Could you check a few things on this drawing? It's one solid part, dimensions in mm from its lowest x, y, z. Coordinates: 2 decimals unless noted, no trailing zeros. Loops run counter-clockwise (first coordinate to the right, second up) from the corner with the lowest first, then second, coordinate; pieces in that order, holes last.
1) Imagine slicing it at B-B on z = 5. Please give me the cut outline in (x, y) (1 decimal).
2) If I drill on line 1 along X through (y, z) = (4.85, 25); line 2 along X through (y, z) = (3.05, 27); line 3 along Z through (x, y) = (44, 1.55) (1 decimal), over which ranges is the centre line in solid material (lowest first)?
3) Will these pins go through, and if not, where does the flat tip stop? P1, Ø6, axis at x = 44, z = 27, coming from the +Y side; P2, Ø6, axis at x = 43, z = 27.71, coming from the +Y side; P3, Ø1, axis at x = 30.5, y = 1, coming from the -Z side; P4, Ø2.5, axis at y = 3, z = 29.5, coming from the -X side (3 decimals).
4) Imagine slicing it at C-C on y = 3. Please give me the cut outline in (x, z), plus the area to 3 significant figures.
5) Imagine slicing it at A-A on x = 43. Please give me the cut outline in (y, z), plus the area to 3 significant figures.
6) Thinking about a two-plate mould opening in X: for the marked faces 1, 2 and 3, which applies, released by +X, released by -X, zero draft, split by the parting line, or undercut?
7) Imagine slicing it at D-D on x = 28. Please give me the cut outline in (y, z).
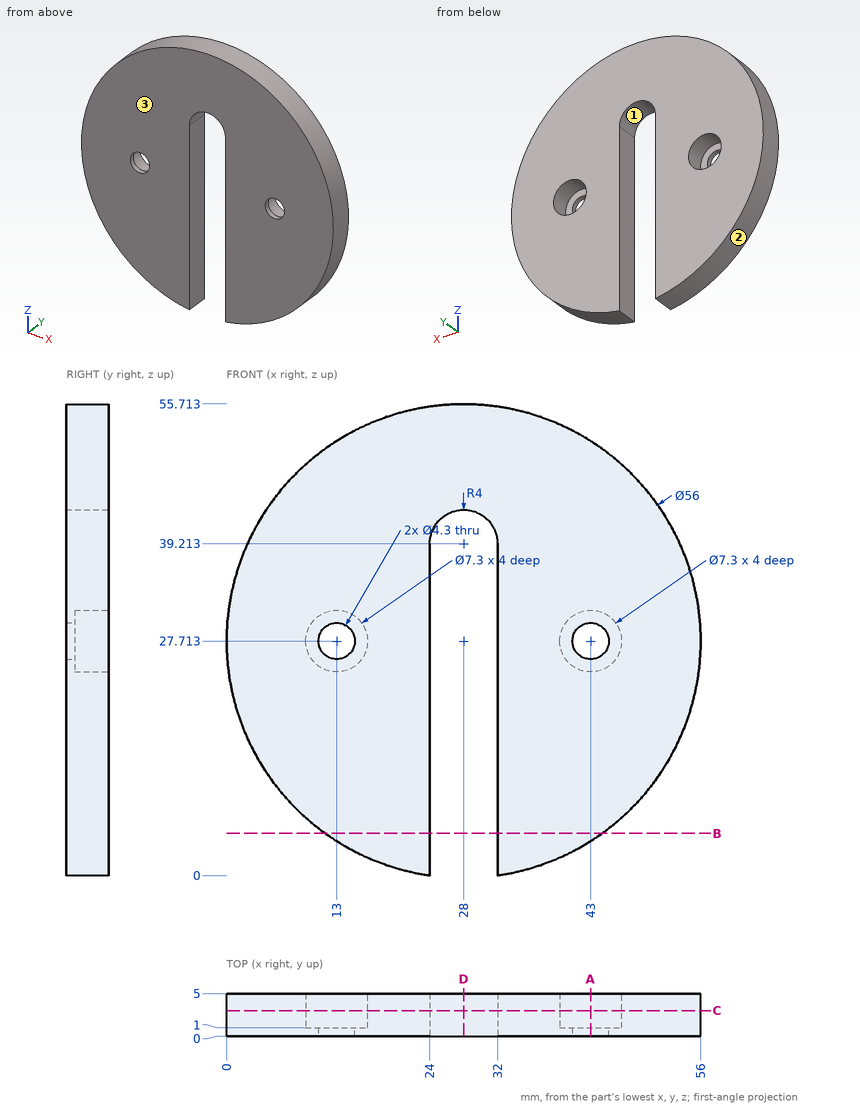
Filled in:
1. outline: (11.6, 0) - (24, 0) - (24, 5) - (11.6, 5) - close; (32, 0) - (44.4, 0) - (44.4, 5) - (32, 5) - close
2. line 1: x = 0.13 to 10.56, 15.44 to 24, 32 to 40.56, 45.44 to 55.87
2. line 2: x = 0.01 to 9.42, 16.58 to 24, 32 to 39.42, 46.58 to 55.99
2. line 3: z = 4.7 to 24.2, 31.2 to 50.7
3. P1: stops at y = 5
3. P2: stops at y = 1
3. P3: stops at z = 41.86
3. P4: stops at x = 0.005
4. outline: (24, 0) - (24, 39.21) arc R4 cw to (32, 39.21) - (32, 0) arc R28 ccw (long way) to start; hole circle Ø7.3 at (13, 27.71); hole circle Ø7.3 at (43, 27.71)
4. area: 2,040 mm2
5. outline: (0, 4.07) - (5, 4.07) - (5, 24.06) - (1, 24.06) - (1, 25.56) - (0, 25.56) - close; (0, 29.86) - (1, 29.86) - (1, 31.36) - (5, 31.36) - (5, 51.36) - (0, 51.36) - close
5. area: 203 mm2
6. face 1: undercut
6. face 2: split by the parting line
6. face 3: zero draft
7. outline: (0, 43.21) - (5, 43.21) - (5, 55.71) - (0, 55.71) - close
